Autodesk Inventor part; units mm, degrees
ref_plane "Work Plane1" through (1.525, 0, 0) normal (0, 0, 1) x (1, 0, 0)
ref_plane "YZ Plane" through (0, 0, 0) normal (1, 0, 0) x (0, 1, 0)
ref_plane "XZ Plane" through (0, 0, 0) normal (0, 1, 0) x (-1, 0, 0)
sketch "Sketch1" plane through (0, 0, 0) normal (0, 0, 1) x (1, 0, 0)
  line L0 (0, 3) -> (16, 3)
  line L1 (16, 3) -> (16, 0)
  line L2 (16, 0) -> (0, 0)
  line L3 (-3.2, 0) -> (19.2, 0)
  line L4 (0, -0.6) -> (0, 3.6)
  line L5 (0, 3) -> (0, 0)
  dimension "d2" = 6
  dimension "d59" = 16
revolve "Body" add sketch "Sketch1" angle 360 about axis through (16, 0, 0) along (-1, 0, 0)
sketch "Sketch2" plane through (0, 0, 0) normal (-1, 0, 0) x (0, 0, 1)
  line L0 (0, 5.7735) -> (5, 2.8868)
  line L1 (5, 2.8868) -> (5, -2.8868)
  line L2 (5, -2.8868) -> (0, -5.7735)
  line L3 (0, -5.7735) -> (-5, -2.8868)
  line L4 (-5, -2.8868) -> (-5, 2.8868)
  line L5 (-5, 2.8868) -> (0, 5.7735)
  line L6 (-7, 0) -> (7, 0)
  line L7 (0, 8.0829) -> (0, -8.0829)
  point P0 (0, 0)
  point P1 (0, 0)
  dimension "d11" = 10
extrude "Head" add sketch "Sketch2" along normal blind 4
sketch "Sketch4" plane through (0, 0, 0) normal (0, 0, 1) x (1, 0, 0)
  line L0 (-3.4226, 6) -> (-4, 5)
  line L1 (-1.1, 0) -> (-0.234, 0)
  line L2 (-4.7532, 0) -> (0.5192, 0)
  line L3 (-4, 6) -> (-3.4226, 6)
  line L4 (-4, 5) -> (-4, 6)
  line L5 (0, 7.2) -> (0, -1.2)
  dimension "d65" = 10
  dimension "d67" = 30
  dimension "d68" = 12
  dimension "d69" = 4
revolve "Chamfer1" cut sketch "Sketch4" angle 360 about axis through (-1.1, 0, 0) along (1, 0, 0)
thread "Thread"
chamfer "Chamfer2" distance 0.6135 distance2 0.6136 1 edges at (16, -3, 0) measured on face at (16, -0.5681, 0.823)
fillet "Fillet2" radius 0.25 1 edges at (0, -3, 0)
ref_plane "Work Plane1" through (1.525, 0, 0) normal (0, 0, 1) x (1, 0, 0)
equation "\"d2\" = GD"
equation "\"d59\" = NLG"
equation "\"d11\" = SW"
equation "\"d3\" = KOH"
equation "\"d71\" = RR"
equation "\"d15\" = GEL"
equation "\"d6\" = -0.5 * SPD + 0.5 * GD"
equation "\"d65\" = SW"
equation "\"d67\" = ANG1"
equation "\"d68\" = 1.2 * SW"
equation "\"d69\" = KOH"
equation "\"NLG\" = 16"
equation "\"GD\" = NND"
equation "\"BDM\" = NND"
equation "\"KOH\" = 4"
equation "\"GEL\" = 15"
equation "\"SW\" = 10"
equation "\"SPD\" = NND - 1.2269 * PTC"
equation "\"SD2\" = NND"
equation "\"SD\" = 0"
equation "\"ANG1\" = 30deg"
equation "\"GAL\" = 0.61345 * PTC"
equation "\"GUL\" = 0.61345 * PTC"
equation "\"RR\" = 0.25"
equation "\"RR1\" = 0.1"
equation "\"WFT\" = 0"
equation "\"GD1\" = THREADDIA - 1.2269 * PTC"
equation "\"THREADDIA\" = 6"
equation "\"TOA\" = 30deg"
equation "\"FAWI\" = 90deg"
equation "\"PTC\" = 1"
equation "\"NND\" = 6"
equation "\"E0\" = 1.155 * SW"
properties part number "Hexagon bolt GB/T 5781 M6 x 16" material "Steel, Mild"
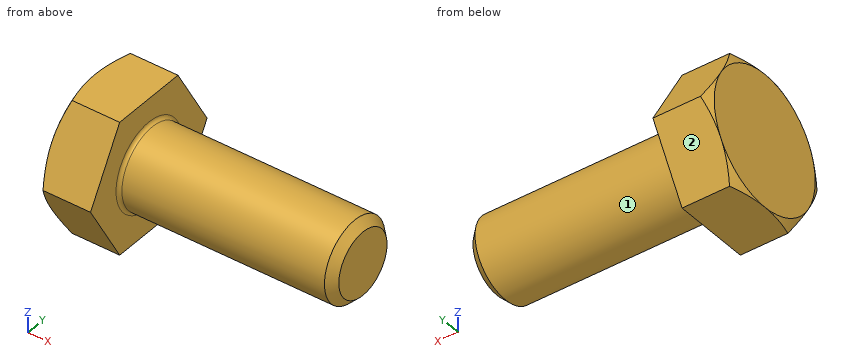
Could you check a few things on this model? Use its own coordinates, in mm. Face numbers are marked on the shaded views. A direction names the side the tool comes from. Give positions to 0.01 mm unless a question says otherwise; leave off trailing zeros. Order: outer loops, then holes, each group sorted by start corner. A loop starts at its lowest first (then second) coordinate and runs counter-clockwise, first axis right, second up. Notation, with made-up numbers: (43, 72.5) -> (87, 72.5) arc R5 cw to (87, 78.5) -> close; hole circle Ø11 at (64, 36.25). An arc over 180 degrees is marked (long way). Answer in a Markdown table with one row per item. Add a question column.
Item 1: For the marked faces 1 and 2, which set-ups out of +Z, -Z, +X, -X, +Y, -Y let a thin tool reach every point of the face, with its end or its side?
Item 2: Imagine slicing it at A-A (x = -0.5). List the corners of the cut face in (y, z) for me.
Item 3: Please list where these lines run through material, in increasing order: probe 1 along X at (y, z) = (-2.25, 4); probe 2 along Y at (x, z) = (3.25, 1.5); probe 3 along Z at (x, y) = (0.5, 0.5).
Item 4: I'm going to push a flat-ended pin straight in: P1, Ø6, axis at x = -1.5, y = -3.5, coming from the +Z side. Where does the tip first touch, or does it pass through?
Item 5: Imagine slicing it at B-B (x = 13). List the corners of the cut face in (y, z) for me.
Result:
| question | item | result |
|---|---|---|
| 1 | face 1 | +X |
| 1 | face 2 | -Z, +X, -X, +Y |
| 2 | outline | (-5.77, 0) -> (-2.89, -5) -> (2.89, -5) -> (5.77, 0) -> (2.89, 5) -> (-2.89, 5) -> close |
| 3 | probe 1 | -4 to 0 |
| 3 | probe 2 | -2.6 to 2.6 |
| 3 | probe 3 | -2.96 to 2.96 |
| 4 | P1 | z = 5 |
| 5 | outline | circle Ø6 at (0, 0) |
